Here's the drawing with two shaded views (mm, measured from the low corner). I have some questions. A direction names the side the tool comes from. Coordinates: 2 decimals unless noted, no trailing zeros. Loops run counter-clockwise (first coordinate to the right, second up) from the corner with the lowest first, then second, coordinate; pieces in that order, holes last.
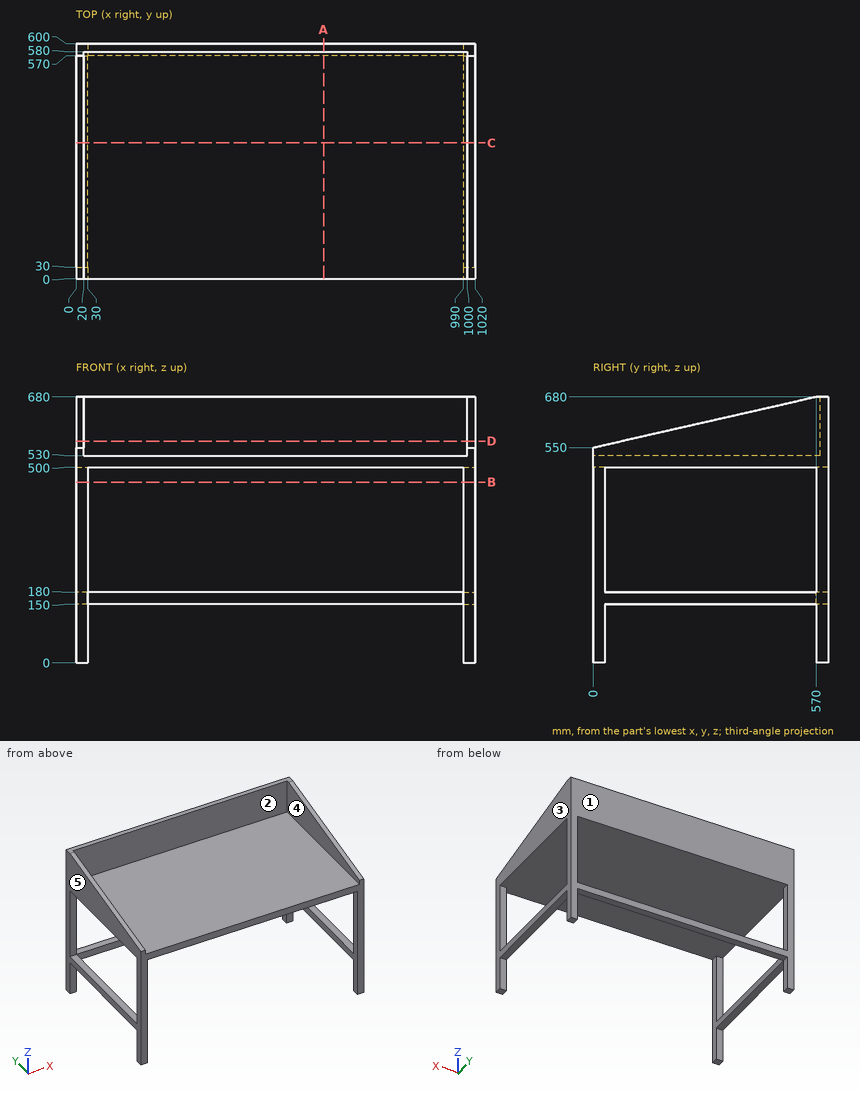
(1) Which directions (+Z, -Z, +X, -X, +Y, -Y) give clear straight access to the entire face, cutting with the end or side of a thin tool? Please do the marked faces 1 and 2.
Check values:
face 1: +Z, -Z, +X, -X, +Y
face 2: +Z, -Y
(2) I want a section at C-C on y = 347.5. Write out the boundary of the cut face in (x, z), then the cut area to 3 significant figures.
Check values:
outline: (0, 150) - (30, 150) - (30, 180) - (0, 180) - close; (0, 500) - (1020, 500) - (1020, 629.25) - (1000, 629.25) - (1000, 530) - (20, 530) - (20, 629.25) - (0, 629.25) - close; (990, 150) - (1020, 150) - (1020, 180) - (990, 180) - close
area: 36,400 mm2
(3) If I drill on probe 1 along X at (y, z) = (517, 637.5); probe 2 along Z at (x, y) = (298, 96.5); probe 3 along Y at (x, z) = (68.5, 607), over which ranges is the centre line in solid material (lowest first)?
Check values:
probe 1: x = 0 to 20, 1000 to 1020
probe 2: z = 500 to 530
probe 3: y = 580 to 600
(4) I want a section at B-B on z = 462. Write out the boundary of the cut face in (x, y).
Check values:
outline: (0, 0) - (30, 0) - (30, 30) - (0, 30) - close; (0, 570) - (30, 570) - (30, 600) - (0, 600) - close; (990, 0) - (1020, 0) - (1020, 30) - (990, 30) - close; (990, 570) - (1020, 570) - (1020, 600) - (990, 600) - close
(5) I want a section at D-D on z = 567. Write out the boundary of the cut face in (x, y).
Check values:
outline: (0, 74.54) - (20, 74.54) - (20, 580) - (1000, 580) - (1000, 74.54) - (1020, 74.54) - (1020, 600) - (0, 600) - close
(6) If we mould it in two halves opening along X, with no side actions, what happens to the marked faces 3, 4 and 5? For each: released by +X, released by -X, zero draft, split by the parting line, or undercut.
Check values:
face 3: released by +X
face 4: undercut
face 5: released by -X
(7) I'm going to push flat-ended pins straight in: pin 1 (24 mm diameter, centred on x = 1004.5, y = 183.5, fed in from -Z); pin 2 (9 mm diameter, centred on x = 16.5, z = 102, fed in from -Y); pin 3 (10 mm diameter, centred on x = 665.5, y = 501.5, fed in from -Z); pin 4 (8 mm diameter, centred on x = 905, z = 535.5, fed in from -Y). Where does each tip first touch, or does it pass through?
Check values:
pin 1: stops at z = 150
pin 2: stops at y = 0
pin 3: stops at z = 500
pin 4: stops at y = 580
(8) I want a section at A-A on x = 633. Write out the boundary of the cut face in (y, z), then the cut area to 3 significant figures.
Check values:
outline: (0, 500) - (600, 500) - (600, 680) - (580, 680) - (580, 530) - (0, 530) - close; (570, 150) - (600, 150) - (600, 180) - (570, 180) - close
area: 21,900 mm2
